For this review, take the finished solid that the model builds, in its own axes (mm). Face numbers are marked on the shaded views. Coordinates: 2 decimals unless noted, no trailing zeros. Loops run counter-clockwise (first coordinate to the right, second up) from the corner with the lowest first, then second, coordinate; pieces in that order, holes last.
1. Take a section at A-A, the plane x = 0. State the section outline as (y, z) points, then the cut area to 3 significant figures.
2. Take a section at B-B, the plane y = 0. State the section outline as (x, z) points, then the cut area to 3 significant figures.
3. Take a section at C-C, the plane z = 1.75. State the section outline as (x, y) points, then the cut area to 3 significant figures.
4. Clearance check with flat-ended pins moving along their axes: P1, Ø3, axis at x = 21, y = 14, coming from the +Z side; P2, Ø8, axis at y = -10.5, z = 11.5, coming from the +X side; P3, Ø3, axis at y = 0.5, z = 11.5, coming from the -X side. State where each tip first meets the part, or that it passes through.
5. To check wall thickness, follow probe 1 along Y at (x, z) = (0, 8.45); probe 2 along Z at (x, y) = (6, -0.5); probe 3 along Z at (x, y) = (26, 22.5). State the ranges of each line that lie inside material, in increasing order.
6. Take a section at D-D, the plane y = -14.5. State the section outline as (x, z) points, then the cut area to 3 significant figures.
7. Mouldability with a two-part tool opening along Y and no side actions: class the marked faces 1, 2 and 3 as pulls with the +Y half, pulls with the -Y half, needs draft (parallel to the pull), parting line crosses it, or undercut.
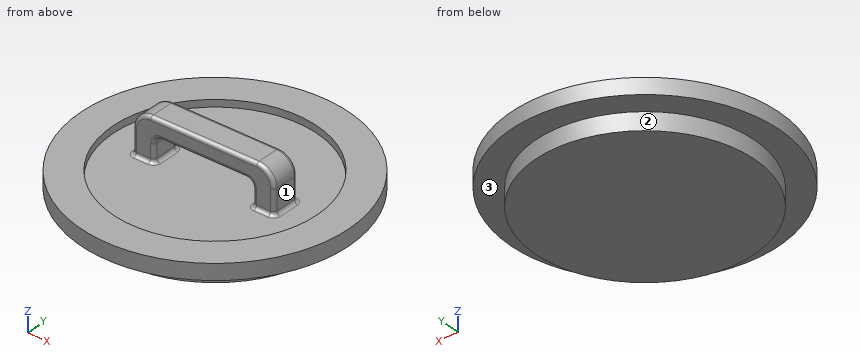
```python
from build123d import *

# Parameters (mm, degrees)
F1_R      = 30.9
F2_DEPTH  = 5
F3_R      = 37.85
F4_DEPTH  = 4.5
F5_R      = 28.85
F6_DEPTH  = 2
F7_W      = 40
F7_H      = 8
F9_DEPTH  = 12
F10_R     = 5
F8_W      = 28
F8_H      = 8
F11_DEPTH = 7
F12_R     = 2
F13_F1_R  = 1
F13_F2_R  = 1


with BuildPart() as f2:
    # F1 (on offset) → F2 (new body)
    with BuildSketch(Plane.XY):
        Circle(F1_R)
    extrude(amount=F2_DEPTH)

    # F3 (on face) → F4 (join)
    with BuildSketch(Plane.XY.offset(5)):
        Circle(F3_R)
    extrude(amount=F4_DEPTH)

    # F5 (on face) → F6 (cut)
    with BuildSketch(Plane.XY.offset(9.5)):
        Circle(F5_R)
    extrude(amount=-F6_DEPTH, mode=Mode.SUBTRACT)

    # F7 (on face) → F9 (join)
    with BuildSketch(Plane.XY.offset(7.5)):
        Rectangle(F7_W, F7_H)
    extrude(amount=F9_DEPTH)

    # F10
    f10_edges = [f2.edges().sort_by_distance(p)[0] for p in [
        (-20, 0, 19.5),
        (20, 0, 19.5),
    ]]
    fillet(f10_edges, radius=F10_R)

    # F8 (on face) → F11 (cut)
    with BuildSketch(Plane.XY.offset(7.5)):
        Rectangle(F8_W, F8_H)
    extrude(amount=F11_DEPTH, mode=Mode.SUBTRACT)

    # F12
    f12_edges = [f2.edges().sort_by_distance(p)[0] for p in [
        (-14, 0, 14.5),
        (14, 0, 14.5),
    ]]
    fillet(f12_edges, radius=F12_R)

    # F13: fillet of radius 1 on 24 edges, made by hand

    # F13_f1
    f13_f1_edges = [f2.edges().sort_by_distance(p)[0] for p in [
        (0, -4, 19.5),
        (14, -4, 10),
        (13.4142135624, -4, 13.9142135624),
        (0, -4, 14.5),
        (-13.4142135624, -4, 13.9142135624),
        (-14, -4, 10),
        (-20, -4, 11),
        (-18.5355339059, -4, 18.0355339059),
        (18.5355339059, -4, 18.0355339059),
        (20, -4, 11),
        (14, 4, 10),
        (13.4142135624, 4, 13.9142135624),
        (0, 4, 14.5),
        (20, 4, 11),
        (-13.4142135624, 4, 13.9142135624),
        (18.5355339059, 4, 18.0355339059),
        (-14, 4, 10),
        (0, 4, 19.5),
        (-18.5355339059, 4, 18.0355339059),
        (-20, 4, 11),
    ]]
    fillet(f13_f1_edges, radius=F13_F1_R)

    # F13_f2
    f13_f2_edges = [f2.edges().sort_by_distance(p)[0] for p in [
        (-17, -4, 7.5),
        (17, -4, 7.5),
        (17, 4, 7.5),
        (-17, 4, 7.5),
        (-14.2928932188, 3.7071067812, 7.5),
        (-19.7071067812, 3.7071067812, 7.5),
        (19.7071067812, 3.7071067812, 7.5),
        (14.2928932188, 3.7071067812, 7.5),
        (14.2928932188, -3.7071067812, 7.5),
        (19.7071067812, -3.7071067812, 7.5),
        (-19.7071067812, -3.7071067812, 7.5),
        (-14.2928932188, -3.7071067812, 7.5),
    ]]
    fillet(f13_f2_edges, radius=F13_F2_R)


solid = f2.part
```
Results list:
1. outline: (-37.85, 5) - (-30.9, 5) - (-30.9, 0) - (30.9, 0) - (30.9, 5) - (37.85, 5) - (37.85, 9.5) - (28.85, 9.5) - (28.85, 7.5) - (-28.85, 7.5) - (-28.85, 9.5) - (-37.85, 9.5) - close; (-4, 15.5) arc R1 ccw to (-3, 14.5) - (3, 14.5) arc R1 ccw to (4, 15.5) - (4, 18.5) arc R1 ccw to (3, 19.5) - (-3, 19.5) arc R1 ccw to (-4, 18.5) - close
1. area: 573 mm2
2. outline: (-37.85, 5) - (-30.9, 5) - (-30.9, 0) - (30.9, 0) - (30.9, 5) - (37.85, 5) - (37.85, 9.5) - (28.85, 9.5) - (28.85, 7.5) - (21, 7.5) arc R1 cw to (20, 8.5) - (20, 14.5) arc R5 ccw to (15, 19.5) - (-15, 19.5) arc R5 ccw to (-20, 14.5) - (-20, 8.5) arc R1 cw to (-21, 7.5) - (-28.85, 7.5) - (-28.85, 9.5) - (-37.85, 9.5) - close; hole (-14, 8.5) arc R1 ccw to (-13, 7.5) - (13, 7.5) arc R1 ccw to (14, 8.5) - (14, 12.5) arc R2 ccw to (12, 14.5) - (-12, 14.5) arc R2 ccw to (-14, 12.5) - close
2. area: 810 mm2
3. outline: circle Ø61.8 at (0, 0)
3. area: 3,000 mm2
4. P1: stops at z = 7.5
4. P2: stops at x = 37.19
4. P3: stops at x = -20
5. probe 1: y = -37.85 to -28.85, 28.85 to 37.85
5. probe 2: z = 0 to 7.5, 14.5 to 19.5
5. probe 3: z = 5 to 9.5
6. outline: (-34.96, 5) - (-27.29, 5) - (-27.29, 0) - (27.29, 0) - (27.29, 5) - (34.96, 5) - (34.96, 9.5) - (24.94, 9.5) - (24.94, 7.5) - (-24.94, 7.5) - (-24.94, 9.5) - (-34.96, 9.5) - close
6. area: 488 mm2
7. face 1: undercut
7. face 2: parting line crosses it
7. face 3: needs draft
